CAD build for the part. Positions are in the model's coordinates, mm. A direction names the side the tool comes from. Coordinates: 2 decimals unless noted, no trailing zeros. Loops run counter-clockwise (first coordinate to the right, second up) from the corner with the lowest first, then second, coordinate; pieces in that order, holes last. Notation, with made-up numbers: (-30, 43) - (-21, 43) arc R9 cw to (-21, 47) - close; hole circle Ø3 at (-28, 6). An arc over 180 degrees is marked (long way). Put each result on its own line as item: value.
```python
from build123d import *

# Parameters (mm, degrees)
BOSS_EXTRUDE1_DEPTH = 3.05
SKETCH2_R           = 1
SKETCH2_R_2         = 1.5
CUT_EXTRUDE1_DEPTH  = 10
FILLET1_R           = 0.5


with BuildPart() as part:
    # Sketch1 → Boss-Extrude1 (new body)
    with BuildSketch(Plane(origin=(0, 0, 0), x_dir=(1, 0, 0), z_dir=(0, 1, 0))):
        Polygon((0, 0), (0, 32.5), (40, 32.5), (40, 0), (32, 0), (34.886751346, -5), (23.386751346, -5), (26.273502692, 0), (13.726497308, 0), (16.613248654, -5), (5.113248654, -5), (8, 0), align=None)
    extrude(amount=BOSS_EXTRUDE1_DEPTH)

    # Sketch2 → Cut-Extrude1 (cut)
    with BuildSketch(Plane(origin=(0, 3.05, 0), x_dir=(1, 0, 0), z_dir=(0, 1, 0))):
        with Locations(Location((8, 30, 0), (0, 0, 270))):
            Circle(SKETCH2_R)
        with Locations(Location((32, 30, 0), (0, 0, 270))):
            Circle(SKETCH2_R)
        with Locations(Location((20, 30, 0), (0, 0, 270))):
            Circle(SKETCH2_R_2)
    extrude(amount=-CUT_EXTRUDE1_DEPTH, mode=Mode.SUBTRACT)

    # Fillet1
    fillet1_edges = [part.edges().sort_by_distance(p)[0] for p in [
        (32, 1.525, 0),
        (34.886751346, 1.525, 5),
        (23.386751346, 1.525, 5),
        (26.273502692, 1.525, 0),
        (13.726497308, 1.525, 0),
        (16.613248654, 1.525, 5),
        (5.113248654, 1.525, 5),
        (8, 1.525, 0),
    ]]
    fillet(fillet1_edges, radius=FILLET1_R)


solid = part.part
```
Q1. Pin check, flat tips, straight feed: pin 1 Ø1.5 at (x, y) = (20.5, 1) entering from +Z; pin 2 Ø1.5 at (x, y) = (35, 2) entering from +Z. Stop position of each tip, or through.
Determined:
pin 1: z = 0
pin 2: z = 4.94
Q2. Slice it at C-C, the plane y = 0.7. Give the cut face in (x, z).
Determined:
outline: (0, -32.5) - (40, -32.5) - (40, 0) - (32.87, 0) arc R0.5 cw to (32.43, 0.75) - (34.45, 4.25) arc R0.5 ccw to (34.02, 5) - (24.25, 5) arc R0.5 ccw to (23.82, 4.25) - (25.84, 0.75) arc R0.5 cw to (25.41, 0) - (14.59, 0) arc R0.5 cw to (14.16, 0.75) - (16.18, 4.25) arc R0.5 ccw to (15.75, 5) - (5.98, 5) arc R0.5 ccw to (5.55, 4.25) - (7.57, 0.75) arc R0.5 cw to (7.13, 0) - (0, 0) - close; hole circle Ø2 at (8, -30); hole circle Ø3 at (20, -30); hole circle Ø2 at (32, -30)
Q3. Tool access for faces 5 (the flat face through (4, 2, 0)), 6 (the flat face through (20, 3.05, -14)), 7 (the flat face through (24.82, 1.5, 2.52)), 8 (the flat face through (40, 2, -16)), 9 (the flat face through (36, 2, 0)): list every direction of +Z, -Z, +X, -X, +Y, -Y with a clear straight run to the whole face (end or side of a thin tool).
Determined:
face 5: -X, +Y, -Y
face 6: +Z, -Z, +X, -X, +Y
face 7: +Y, -Y
face 8: +Z, -Z, +X, +Y, -Y
face 9: +X, +Y, -Y
Q4. Mould opens along Z. For faces 1 (the flat face through (29, 2, 5)), 2 (the flat face through (20, 2, 0)), 3 (the flat face through (20, 2, -32.5)), 4 (the flat face through (20, 0, -14)) say: +Z half, -Z half, draft (parallel to the pull), parting line (faces both ways), or undercut.
Determined:
face 1: +Z half
face 2: undercut
face 3: -Z half
face 4: draft
Q5. Wall check: L1, parallel to X at y = 1.2, z = -30; L2, parallel to Z at x = 16.5, y = 2.9. Give the ranges that are in metal, low to high. Write a range as from..to.
Determined:
L1: 0..7, 9..18.5, 21.5..31, 33..40
L2: -32.5..0
Q6. Slice it at A-A, the plane x = 20. Give the cut face in (y, z), then the cut area to 3 significant figures.
Determined:
outline: (0, -32.5) - (3.05, -32.5) - (3.05, -31.5) - (0, -31.5) - close; (0, -28.5) - (3.05, -28.5) - (3.05, 0) - (0, 0) - close
area: 90.0 mm2
Q7. Slice it at B-B, the plane z = -30. Give the cut face in (x, y).
Determined:
outline: (0, 0) - (7, 0) - (7, 3.05) - (0, 3.05) - close; (9, 0) - (18.5, 0) - (18.5, 3.05) - (9, 3.05) - close; (21.5, 0) - (31, 0) - (31, 3.05) - (21.5, 3.05) - close; (33, 0) - (40, 0) - (40, 3.05) - (33, 3.05) - close
